from build123d import *

# Parameters (mm, degrees)
BOSS_EXTRUDE1_DEPTH      = 2.54
SKETCH5_W                = 10.06
SKETCH5_H                = 1.5
CUT_EXTRUDE3_DEPTH       = 0.7
SKETCH3_W                = 0.64
SKETCH3_H                = 0.64
CUT_EXTRUDE2_DEPTH       = 3.54
SKETCH4_W                = 0.64
SKETCH4_H                = 0.64
BOSS_EXTRUDE2_DEPTH      = 8.2
BOSS_EXTRUDE2_DEPTH_BACK = 2.8
CHAMFER1_SIZE            = 0.16
CHAMFER1_SIZE2           = 0.5458
CHAMFER1_PART_2_SIZE     = 0.16
CHAMFER1_PART_2_SIZE2    = 0.5458
CHAMFER1_PART_3_SIZE     = 0.16
CHAMFER1_PART_3_SIZE2    = 0.5458
CHAMFER1_PART_4_SIZE     = 0.16
CHAMFER1_PART_4_SIZE2    = 0.5458
CHAMFER2_SIZE            = 0.16
CHAMFER2_SIZE2           = 0.5458
CHAMFER2_PART_2_SIZE     = 0.16
CHAMFER2_PART_2_SIZE2    = 0.5458
CHAMFER2_PART_3_SIZE     = 0.16
CHAMFER2_PART_3_SIZE2    = 0.5458
CHAMFER2_PART_4_SIZE     = 0.16
CHAMFER2_PART_4_SIZE2    = 0.5458


with BuildPart() as part:
    # Sketch1 → Boss-Extrude1 (new body)
    with BuildSketch(Plane(origin=(0, 0, 0), x_dir=(1, 0, 0), z_dir=(0, 1, 0))):
        Polygon((-4.660019462, -1.25), (-3.034980538, -1.25), (-2.665, -0.75), (-2.465, -0.75), (-2.095019462, -1.25), (-0.469980538, -1.25), (-0.1, -0.75), (0.1, -0.75), (0.469980538, -1.25), (2.095019462, -1.25), (2.465, -0.75), (2.665, -0.75), (3.034980538, -1.25), (4.660019462, -1.25), (5.03, -0.75), (5.03, 0.75), (4.660019462, 1.25), (3.034980538, 1.25), (2.665, 0.75), (2.465, 0.75), (2.095019462, 1.25), (0.469980538, 1.25), (0.1, 0.75), (-0.1, 0.75), (-0.469980538, 1.25), (-2.095019462, 1.25), (-2.465, 0.75), (-2.665, 0.75), (-3.034980538, 1.25), (-4.660019462, 1.25), (-5.03, 0.75), (-5.03, -0.75), align=None)
    extrude(amount=-BOSS_EXTRUDE1_DEPTH)

    # Sketch5 → Cut-Extrude3 (cut)
    with BuildSketch(Plane(origin=(0, 0, 0), x_dir=(1, 0, 0), z_dir=(0, 1, 0))):
        Rectangle(SKETCH5_W, SKETCH5_H)
    extrude(amount=-CUT_EXTRUDE3_DEPTH, mode=Mode.SUBTRACT)

    # Sketch3 → Cut-Extrude2 (cut, through all)
    with BuildSketch(Plane(origin=(0, -2.54, 0), x_dir=(-1, 0, 0), z_dir=(0, -1, 0))):
        with Locations((-3.81, 0)):
            Rectangle(SKETCH3_W, SKETCH3_H)
        with Locations((-1.27, 0)):
            Rectangle(SKETCH3_W, SKETCH3_H)
        with Locations((1.27, 0)):
            Rectangle(SKETCH3_W, SKETCH3_H)
        with Locations((3.81, 0)):
            Rectangle(SKETCH3_W, SKETCH3_H)
    extrude(amount=-CUT_EXTRUDE2_DEPTH, mode=Mode.SUBTRACT)

    # Sketch4 → Boss-Extrude2 (add, two sides)
    with BuildSketch(Plane.XZ) as boss_extrude2_sk:
        with Locations((3.81, 0)):
            Rectangle(SKETCH4_W, SKETCH4_H)
        with Locations((1.27, 0)):
            Rectangle(SKETCH4_W, SKETCH4_H)
        with Locations((-1.27, 0)):
            Rectangle(SKETCH4_W, SKETCH4_H)
        with Locations((-3.81, 0)):
            Rectangle(SKETCH4_W, SKETCH4_H)
    extrude(amount=BOSS_EXTRUDE2_DEPTH)
    extrude(boss_extrude2_sk.sketch, amount=-BOSS_EXTRUDE2_DEPTH_BACK)

    # Chamfer1
    chamfer1_edges = [part.edges().sort_by_distance(p)[0] for p in [
        (3.49, -8.2, 0),
        (3.81, -8.2, -0.32),
        (4.13, -8.2, 0),
        (3.81, -8.2, 0.32),
    ]]
    chamfer1_side = [part.faces().sort_by_distance(p)[0] for p in [
        (3.81, -8.2, 0),
    ]]
    chamfer(chamfer1_edges, length=CHAMFER1_SIZE, length2=CHAMFER1_SIZE2, reference=chamfer1_side[0])

    # Chamfer1 part 2
    chamfer1_part_2_edges = [part.edges().sort_by_distance(p)[0] for p in [
        (0.95, -8.2, 0),
        (1.27, -8.2, -0.32),
        (1.59, -8.2, 0),
        (1.27, -8.2, 0.32),
    ]]
    chamfer1_part_2_side = [part.faces().sort_by_distance(p)[0] for p in [
        (1.27, -8.2, 0),
    ]]
    chamfer(chamfer1_part_2_edges, length=CHAMFER1_PART_2_SIZE, length2=CHAMFER1_PART_2_SIZE2, reference=chamfer1_part_2_side[0])

    # Chamfer1 part 3
    chamfer1_part_3_edges = [part.edges().sort_by_distance(p)[0] for p in [
        (-1.59, -8.2, 0),
        (-1.27, -8.2, -0.32),
        (-0.95, -8.2, 0),
        (-1.27, -8.2, 0.32),
    ]]
    chamfer1_part_3_side = [part.faces().sort_by_distance(p)[0] for p in [
        (-1.27, -8.2, 0),
    ]]
    chamfer(chamfer1_part_3_edges, length=CHAMFER1_PART_3_SIZE, length2=CHAMFER1_PART_3_SIZE2, reference=chamfer1_part_3_side[0])

    # Chamfer1 part 4
    chamfer1_part_4_edges = [part.edges().sort_by_distance(p)[0] for p in [
        (-4.13, -8.2, 0),
        (-3.81, -8.2, -0.32),
        (-3.49, -8.2, 0),
        (-3.81, -8.2, 0.32),
    ]]
    chamfer1_part_4_side = [part.faces().sort_by_distance(p)[0] for p in [
        (-3.81, -8.2, 0),
    ]]
    chamfer(chamfer1_part_4_edges, length=CHAMFER1_PART_4_SIZE, length2=CHAMFER1_PART_4_SIZE2, reference=chamfer1_part_4_side[0])

    # Chamfer2
    chamfer2_edges = [part.edges().sort_by_distance(p)[0] for p in [
        (3.49, 2.8, 0),
        (3.81, 2.8, -0.32),
        (4.13, 2.8, 0),
        (3.81, 2.8, 0.32),
    ]]
    chamfer2_side = [part.faces().sort_by_distance(p)[0] for p in [
        (3.81, 2.8, 0),
    ]]
    chamfer(chamfer2_edges, length=CHAMFER2_SIZE, length2=CHAMFER2_SIZE2, reference=chamfer2_side[0])

    # Chamfer2 part 2
    chamfer2_part_2_edges = [part.edges().sort_by_distance(p)[0] for p in [
        (0.95, 2.8, 0),
        (1.27, 2.8, -0.32),
        (1.59, 2.8, 0),
        (1.27, 2.8, 0.32),
    ]]
    chamfer2_part_2_side = [part.faces().sort_by_distance(p)[0] for p in [
        (1.27, 2.8, 0),
    ]]
    chamfer(chamfer2_part_2_edges, length=CHAMFER2_PART_2_SIZE, length2=CHAMFER2_PART_2_SIZE2, reference=chamfer2_part_2_side[0])

    # Chamfer2 part 3
    chamfer2_part_3_edges = [part.edges().sort_by_distance(p)[0] for p in [
        (-1.59, 2.8, 0),
        (-1.27, 2.8, -0.32),
        (-0.95, 2.8, 0),
        (-1.27, 2.8, 0.32),
    ]]
    chamfer2_part_3_side = [part.faces().sort_by_distance(p)[0] for p in [
        (-1.27, 2.8, 0),
    ]]
    chamfer(chamfer2_part_3_edges, length=CHAMFER2_PART_3_SIZE, length2=CHAMFER2_PART_3_SIZE2, reference=chamfer2_part_3_side[0])

    # Chamfer2 part 4
    chamfer2_part_4_edges = [part.edges().sort_by_distance(p)[0] for p in [
        (-4.13, 2.8, 0),
        (-3.81, 2.8, -0.32),
        (-3.49, 2.8, 0),
        (-3.81, 2.8, 0.32),
    ]]
    chamfer2_part_4_side = [part.faces().sort_by_distance(p)[0] for p in [
        (-3.81, 2.8, 0),
    ]]
    chamfer(chamfer2_part_4_edges, length=CHAMFER2_PART_4_SIZE, length2=CHAMFER2_PART_4_SIZE2, reference=chamfer2_part_4_side[0])


solid = part.part
Design review of the part built by this model. Coordinates are the model's own, in mm. Coordinates: 2 decimals unless noted, no trailing zeros. Loops run counter-clockwise (first coordinate to the right, second up) from the corner with the lowest first, then second, coordinate; pieces in that order, holes last. Notation, with made-up numbers: M 17.5,70 L 43.5,70 A23 ccw 43.5,98 Z; hole C -13,-17 d9. An arc over 180 degrees is marked long. Use one line per item in the form item = value.
(1) For line 1 along X through (y, z) = (-3.25, 0.25); line 2 along Y through (x, z) = (4.25, 0.95), list the stretches that pass through material, from the lowest coordinate up. Write a range as from..to.
Return value:
line_1 = -4.13..-3.49, -1.59..-0.95, 0.95..1.59, 3.49..4.13
line_2 = -2.54..0
(2) Consider section D-D (z = -0.6). Write out the cut boundary in (x, y).
Return value:
outline = M -5.03,-2.54 L 5.03,-2.54 L 5.03,-0.7 L -5.03,-0.7 Z
(3) Consider section B-B (z = 1.1). Write out the cut boundary in (x, y).
Return value:
outline = M -4.77,-2.54 L -2.92,-2.54 L -2.92,0 L -4.77,0 Z; M -2.21,-2.54 L -0.36,-2.54 L -0.36,0 L -2.21,0 Z; M 0.36,-2.54 L 2.21,-2.54 L 2.21,0 L 0.36,0 Z; M 2.92,-2.54 L 4.77,-2.54 L 4.77,0 L 2.92,0 Z
(4) Clearance check with flat-ended pins moving along their axes: P1, Ø0.5, axis at y = -5.5, z = 0, coming from the -X side; P2, Ø0.7, axis at x = -3.5, y = -5, coming from the -Z side. State where each tip first meets the part, or that it passes through.
Return value:
P1 = -4.13
P2 = -0.32
(5) Draft analysis for pull direction X (two halves, no side actions). For faces 1 (the face through (5.03, -2, 0)), 2 (the face through (0, -0.7, 0)), 3 (the face through (-4, -1, -1.25)), 4 (the face through (0, -2.54, 0)), state which applies: pulls with the +X half, pulls with the -X half, needs draft (parallel to the pull), parting line crosses it, or undercut.
Return value:
face_1 = pulls with the +X half
face_2 = undercut
face_3 = needs draft
face_4 = undercut
(6) Consider section A-A (y = -7.25). Write out the cut boundary in (x, z).
Return value:
outline = M -4.13,-0.32 L -3.49,-0.32 L -3.49,0.32 L -4.13,0.32 Z; M -1.59,-0.32 L -0.95,-0.32 L -0.95,0.32 L -1.59,0.32 Z; M 0.95,-0.32 L 1.59,-0.32 L 1.59,0.32 L 0.95,0.32 Z; M 3.49,-0.32 L 4.13,-0.32 L 4.13,0.32 L 3.49,0.32 Z
